from build123d import *

# Parameters (mm, degrees)
F0_R     = 4.55
F1_DEPTH = 25
F2_R     = 3.715
F3_DEPTH = 5
F4_R     = 3.02
F5_DEPTH = 3.45
F6_R     = 1.25
F7_DEPTH = 1
F8_R     = 1.85
F8_R_2   = 1.25
F9_DEPTH = 2.8


with BuildPart() as f1:
    # F0 (on Top) → F1 (new body)
    with BuildSketch(Plane.XY):
        Circle(F0_R)
    extrude(amount=F1_DEPTH)

    # F2 (on face) → F3 (join)
    with BuildSketch(Plane.XY.offset(25)):
        Circle(F2_R)
    extrude(amount=F3_DEPTH)

    # F4 (on face) → F5 (join)
    with BuildSketch(Plane.XY.offset(30)):
        Circle(F4_R)
    extrude(amount=F5_DEPTH)

    # F6 (on face) → F7 (join)
    with BuildSketch(Plane.XY.offset(33.45)):
        Circle(F6_R)
    extrude(amount=F7_DEPTH)

    # F8 (on face) → F9 (join)
    with BuildSketch(Plane.XY.offset(34.45)):
        Circle(F8_R)
        Circle(F8_R_2, mode=Mode.SUBTRACT)
        Circle(F8_R_2)
    extrude(amount=F9_DEPTH)


solid = f1.part
Source: CAD feature listing. Evaluate the final solid. Frame: model axes, mm. A direction names the side the tool comes from. Coordinates: 2 decimals unless noted, no trailing zeros. Write each loop counter-clockwise with the first axis right and the second up, starting at its lowest first coordinate (ties: lowest second). Pieces come first, ordered by that corner, then holes. Notation, with made-up numbers: M -24.75,20.5 L -10.75,20.5 A24 ccw -10.75,47.5 Z; hole C 66,19 d4. An arc over 180 degrees is marked long. Use a Markdown table: item, result.
1) Mould query, pull axis Z, two halves, no side actions, for faces 3 (the flat face through (1, -1, 33.45)), 4 (the cylindrical face through (-0.27, -1.22, 33.94)), 5 (the flat face through (-4, 0, 25)), 6 (the cylindrical face through (-0.99, -4.44, 12.32)). Classes: pulls with the +Z half, pulls with the -Z half, needs draft (parallel to the pull), parting line crosses it, or undercut.
Conclusion:
| item | result |
|---|---|
| face 3 | undercut |
| face 4 | undercut |
| face 5 | pulls with the +Z half |
| face 6 | needs draft |
2) Section C-C, the plane z = 22.5. Output: boundary loops of the cut face in (x, y).
Conclusion:
| item | result |
|---|---|
| outline | C 0,0 d9.1 |
3) Section A-A, the plane y = 0. Output: boundary loops of the cut face in (x, z) (3 decimals).
Conclusion:
| item | result |
|---|---|
| outline | M -4.55,0 L 4.55,0 L 4.55,25 L 3.715,25 L 3.715,30 L 3.02,30 L 3.02,33.45 L 1.25,33.45 L 1.25,34.45 L 1.85,34.45 L 1.85,37.25 L -1.85,37.25 L -1.85,34.45 L -1.25,34.45 L -1.25,33.45 L -3.02,33.45 L -3.02,30 L -3.715,30 L -3.715,25 L -4.55,25 Z |
4) Section D-D, the plane x = 2.5. Output: boundary loops of the cut face in (y, z).
Conclusion:
| item | result |
|---|---|
| outline | M -3.8,0 L 3.8,0 L 3.8,25 L 2.75,25 L 2.75,30 L 1.69,30 L 1.69,33.45 L -1.69,33.45 L -1.69,30 L -2.75,30 L -2.75,25 L -3.8,25 Z |
5) Reachability of faces 1 (the flat face through (0, 0, 0)), 2 (the cylindrical face through (-0.393, 2.994, 31.701)) from +Z, -Z, +X, -X, +Y, -Y: full face, straight path, thin tool, end or side. Return the list, or none.
Conclusion:
| item | result |
|---|---|
| face 1 | -Z, +X, -X, +Y, -Y |
| face 2 | +Z |
6) First-contact query: pin 1 Ø2 at (x, z) = (2, 16) entering from -Y; pin 2 Ø1.5 at (x, z) = (2.5, 22.5) entering from -Y; pin 3 Ø2 at (y, z) = (-2.5, 5) entering from -X. Flat tips, straight axial feed; report the tip coordinate or a pass-through.
Conclusion:
| item | result |
|---|---|
| pin 1 | stops at y = -4.44 |
| pin 2 | stops at y = -4.2 |
| pin 3 | stops at x = -4.3 |
7) Ray query, L1, parallel to Z at x = -1.5, y = 0.25; L2, parallel to Z at x = -0.25, y = -2; L3, parallel to Y at x = 0.25, z = 8. Return the intervals inside material, ascending.
Conclusion:
| item | result |
|---|---|
| L1 | z = 0 to 33.45, 34.45 to 37.25 |
| L2 | z = 0 to 33.45 |
| L3 | y = -4.54 to 4.54 |
